Here's the drawing with two shaded views (mm, measured from the low corner). I have some questions. A direction names the side the tool comes from. Coordinates: 2 decimals unless noted, no trailing zeros. Loops run counter-clockwise (first coordinate to the right, second up) from the corner with the lowest first, then second, coordinate; pieces in that order, holes last. Notation, with made-up numbers: (-2, 66.25) - (35, 66.25) arc R30 ccw to (35, 94.25) - close; hole circle Ø5 at (63, 20). An arc over 180 degrees is marked (long way). One line per item, written item: value. Start each with the question number.
(1) If I drill on line 1 along X through (y, z) = (49, 57); line 2 along Z through (x, y) = (38, 53); line 3 along Z through (x, y) = (54.5, 59), over which ranges is the centre line in solid material (lowest first)? Write a range as from..to.
(2) If we section it at B-B on z = 57.15: Write out the boundary of the cut face in (x, y) (3 decimals).
(3) If we section it at C-C on x = 63.5: Write out the boundary of the cut face in (y, z) (3 decimals), then the cut area to 3 significant figures.
(4) I'm going to push flat-ended pins straight in: P1, Ø10, axis at y = 53, z = 55, coming from the +X side; P2, Ø14, axis at y = 49.5, z = 38, coming from the -X side; P3, Ø2, axis at x = 88, z = 72.5, coming from the +Y side. Where does each tip first touch, or does it pass through?
(5) On a 3-axis mill with a long thin cutter (end or side, diameter ignored), from which of +Z, -Z, +X, -X, +Y, -Y can I reach the whole of each face in a straight line? I mean the marked faces 1, 2 and 3. Say none if no direction works.
(6) If we section it at A-A on y = 46.5: Write out the boundary of the cut face in (x, z) (3 decimals), then the cut area to 3 significant figures.
(7) If we section it at D-D on x = 44: Write out the boundary of the cut face in (y, z), then the cut area to 3 significant figures.
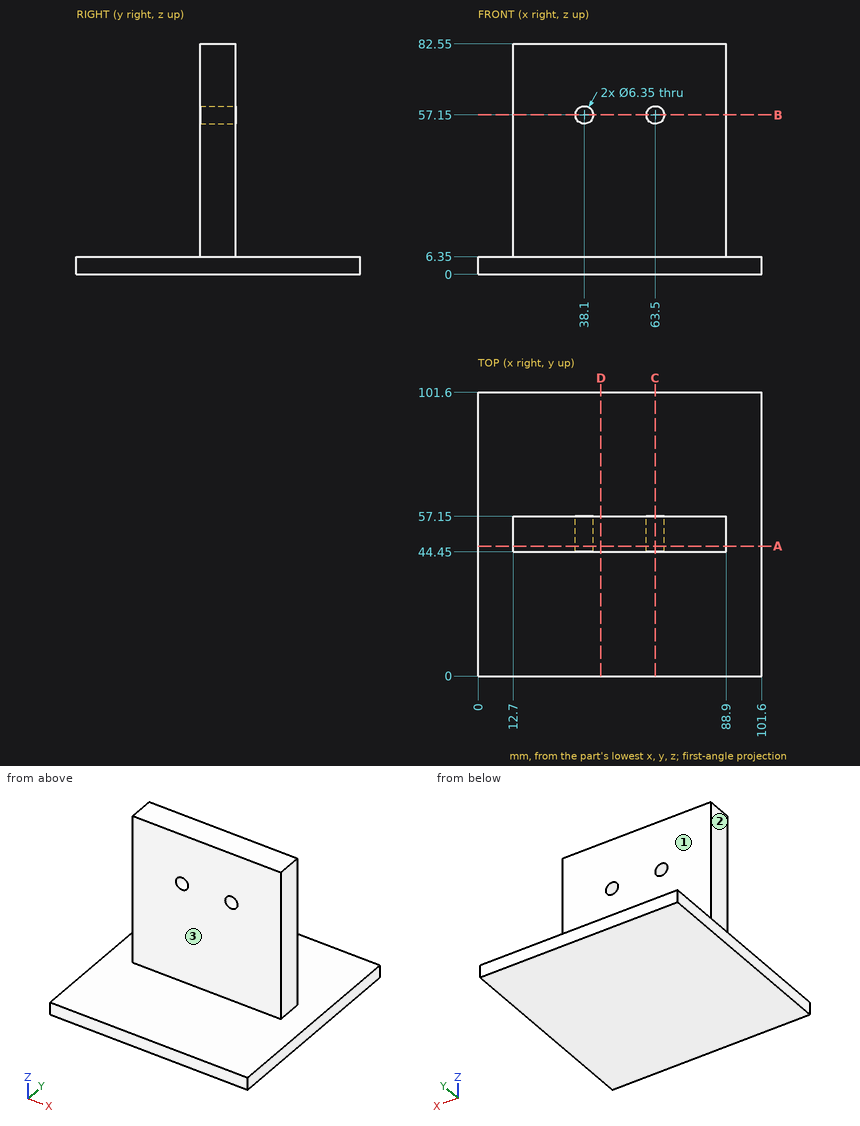
Values:
1. line 1: x = 12.7..34.93, 41.27..60.33, 66.67..88.9
1. line 2: z = 0..53.98, 60.32..82.55
1. line 3: z = 0..6.35
2. outline: (12.7, 44.45) - (34.925, 44.45) - (34.925, 57.15) - (12.7, 57.15) - close; (41.275, 44.45) - (60.325, 44.45) - (60.325, 57.15) - (41.275, 57.15) - close; (66.675, 44.45) - (88.9, 44.45) - (88.9, 57.15) - (66.675, 57.15) - close
3. outline: (0, 0) - (101.6, 0) - (101.6, 6.35) - (57.15, 6.35) - (57.15, 53.975) - (44.45, 53.975) - (44.45, 6.35) - (0, 6.35) - close; (44.45, 60.325) - (57.15, 60.325) - (57.15, 82.55) - (44.45, 82.55) - close
3. area: 1,530 mm2
4. P1: stops at x = 88.9
4. P2: stops at x = 12.7
4. P3: stops at y = 57.15
5. face 1: +Z, +X, -X, +Y
5. face 2: +Z, -X, +Y, -Y
5. face 3: +Z, +X, -X, -Y
6. outline: (0, 0) - (101.6, 0) - (101.6, 6.35) - (88.9, 6.35) - (88.9, 82.55) - (12.7, 82.55) - (12.7, 6.35) - (0, 6.35) - close; hole circle Ø6.35 at (38.1, 57.15); hole circle Ø6.35 at (63.5, 57.15)
6. area: 6,390 mm2
7. outline: (0, 0) - (101.6, 0) - (101.6, 6.35) - (57.15, 6.35) - (57.15, 82.55) - (44.45, 82.55) - (44.45, 6.35) - (0, 6.35) - close
7. area: 1,610 mm2
